Here's the drawing with two shaded views (mm, measured from the low corner). I have some questions. Coordinates: 2 decimals unless noted, no trailing zeros. Write each loop counter-clockwise with the first axis right and the second up, starting at its lowest first coordinate (ties: lowest second). Pieces come first, ordered by that corner, then holes.
Item 1: If we section it at D-D (x = 155.5): Please give me the cut outline in (y, z) (1 decimal), then the cut area to 3 significant figures.
Item 2: If we section it at A-A (y = 483): Please give me the cut outline in (x, z) (1 decimal).
Item 3: I'm going to push flat-ended pins straight in: pin 1 Ø4 at (y, z) = (326, 5.5) entering from -X (1 decimal); pin 2 Ø6.5 at (x, z) = (161.5, 9) entering from -Y (1 decimal). Where does each tip first touch, or does it pass through?
Item 4: If we section it at B-B (x = 193.5): Count the separate pieces of the cut face and the enclosed holes in it.
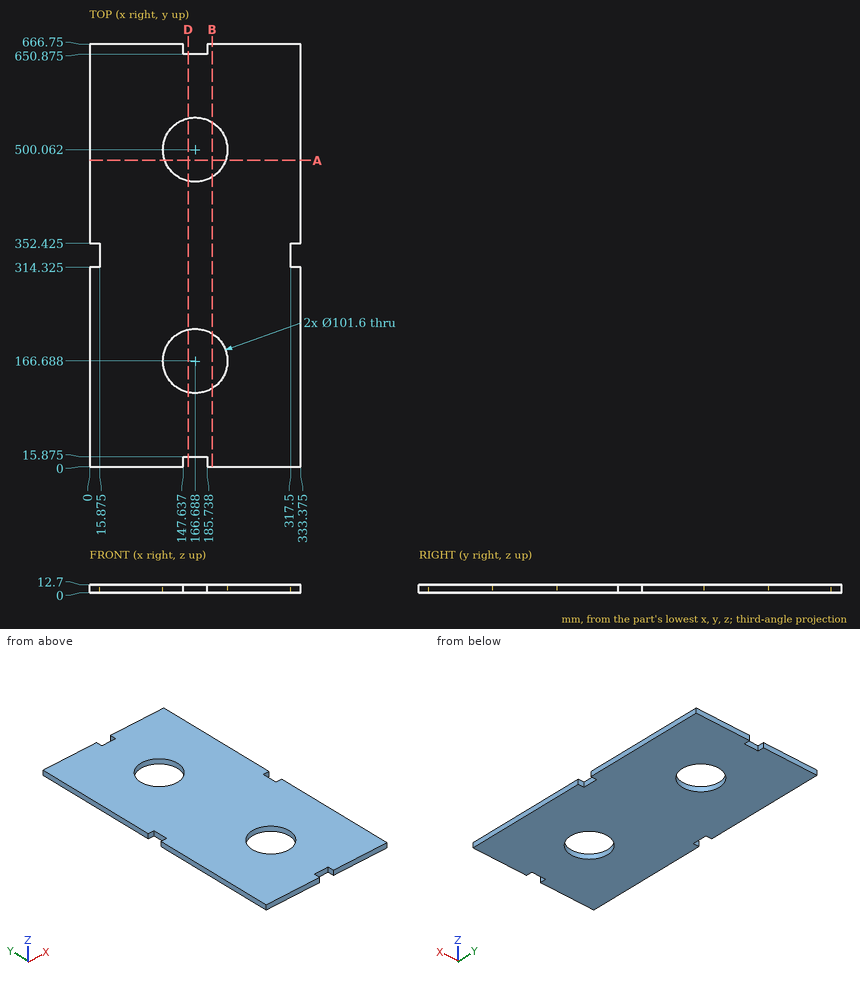
Answer list:
1. outline: (15.9, 0) - (117.1, 0) - (117.1, 12.7) - (15.9, 12.7) - close; (216.2, 0) - (450.5, 0) - (450.5, 12.7) - (216.2, 12.7) - close; (549.6, 0) - (650.9, 0) - (650.9, 12.7) - (549.6, 12.7) - close
1. area: 5,550 mm2
2. outline: (0, 0) - (118.8, 0) - (118.8, 12.7) - (0, 12.7) - close; (214.5, 0) - (333.4, 0) - (333.4, 12.7) - (214.5, 12.7) - close
3. pin 1: stops at x = 15.9
3. pin 2: stops at y = 15.9
4. separate pieces: 3
4. enclosed holes: 0
